Work out the finished part from the listing and answer in its coordinate system (mm). Face numbers are marked on the shaded views. A direction names the side the tool comes from. Give positions to 0.01 mm unless a question says otherwise; leave off trailing zeros. Order: outer loops, then holes, each group sorted by start corner. A loop starts at its lowest first (then second) coordinate and runs counter-clockwise, first axis right, second up.
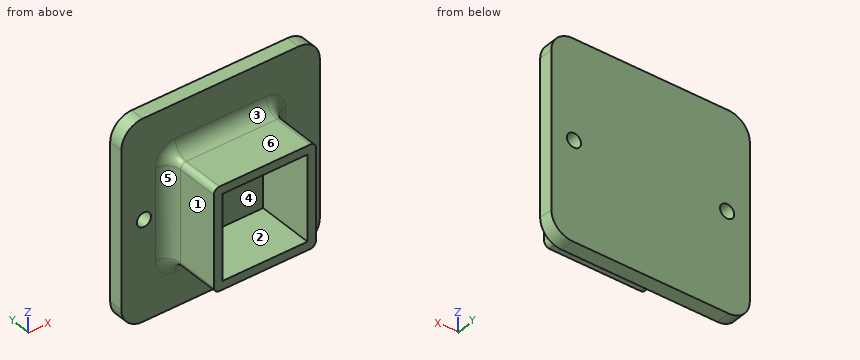
```python
from build123d import *

# Parameters (mm, degrees)
SKETCH1_W           = 36
SKETCH1_H           = 36
SKETCH1_W_2         = 30.02
SKETCH1_H_2         = 30.02
BOSS_EXTRUDE1_DEPTH = 20
SKETCH2_W           = 70
SKETCH2_H           = 70
BOSS_EXTRUDE2_DEPTH = 5
FILLET1_R           = 7.5
SKETCH3_R           = 2.5
CUT_EXTRUDE1_DEPTH  = 56.452682532
FILLET2_R           = 2
FILLET3_R           = 5


with BuildPart() as part:
    # Sketch1 → Boss-Extrude1 (new body)
    with BuildSketch(Plane(origin=(0, 0, 0), x_dir=(1, 0, 0), z_dir=(0, 1, 0))):
        Rectangle(SKETCH1_W, SKETCH1_H)
        Rectangle(SKETCH1_W_2, SKETCH1_H_2, mode=Mode.SUBTRACT)
    extrude(amount=BOSS_EXTRUDE1_DEPTH)

    # Sketch2 → Boss-Extrude2 (add)
    with BuildSketch(Plane(origin=(0, 20, 0), x_dir=(1, 0, 0), z_dir=(0, 1, 0))):
        Rectangle(SKETCH2_W, SKETCH2_H)
    extrude(amount=BOSS_EXTRUDE2_DEPTH)

    # Fillet1
    fillet1_edges = [part.edges().sort_by_distance(p)[0] for p in [
        (35, 22.5, 35),
        (35, 22.5, -35),
        (-35, 22.5, -35),
        (-35, 22.5, 35),
    ]]
    fillet(fillet1_edges, radius=FILLET1_R)

    # Sketch3 → Cut-Extrude1 (cut, through all)
    with BuildSketch(Plane(origin=(0, 25, 0), x_dir=(1, 0, 0), z_dir=(0, 1, 0))):
        with Locations(Location((-27, 0, 0), (0, 0, 270))):
            Circle(SKETCH3_R)
        with Locations(Location((27, 0, 0), (0, 0, 270))):
            Circle(SKETCH3_R)
    extrude(amount=-CUT_EXTRUDE1_DEPTH, mode=Mode.SUBTRACT)

    # Fillet2
    fillet2_edges = [part.edges().sort_by_distance(p)[0] for p in [
        (18, 10, 18),
        (-18, 10, 18),
        (-18, 10, -18),
        (18, 10, -18),
    ]]
    fillet(fillet2_edges, radius=FILLET2_R)

    # Fillet3
    fillet3_edges = [part.edges().sort_by_distance(p)[0] for p in [
        (0, 20, -18),
        (18, 20, 0),
        (0, 20, 18),
        (-18, 20, 0),
        (17.414213562, 20, -17.414213562),
        (17.414213562, 20, 17.414213562),
        (-17.414213562, 20, -17.414213562),
        (-17.414213562, 20, 17.414213562),
    ]]
    fillet(fillet3_edges, radius=FILLET3_R)


solid = part.part
```
1. The part is cut by section D-D (x = 4.5). Write down the section's boundary in (y, z), then the cut area to 3 significant figures.
Findings below:
outline: (0, -18) - (15, -18) arc R5 cw to (20, -23) - (20, -35) - (25, -35) - (25, 35) - (20, 35) - (20, 23) arc R5 cw to (15, 18) - (0, 18) - (0, 15.01) - (20, 15.01) - (20, -15.01) - (0, -15.01) - close
area: 480 mm2
2. Straight lines are drawn through the part: probe 1 along X at (y, z) = (22.65, 0); probe 2 along Z at (x, y) = (-6.5, 4.75). For each, find the intervals that lie inside material, in ascending order.
Findings below:
probe 1: x = -35 to -29.5, -24.5 to 24.5, 29.5 to 35
probe 2: z = -18 to -15.01, 15.01 to 18
3. The mould has two halves that part along Z. Classify the marked faces 1, 2 and 3: pulls with the +Z half, pulls with the -Z half, needs draft (parallel to the pull), parting line crosses it, or undercut.
Findings below:
face 1: needs draft
face 2: undercut
face 3: pulls with the +Z half
4. Which of the six approach directions +Z, -Z, +X, -X, +Y, -Y give full straight-line access (tool end or side, diameter ignored) to the marked faces 4, 5 and 6?
Findings below:
face 4: -Y
face 5: +Z, -Z, -X, -Y
face 6: +Z, +X, -X, -Y
5. The part is cut by section B-B (y = 10.5). Write down the section's boundary in (x, z), then the cut area to 3 significant figures.
Findings below:
outline: (-18, -16) arc R2 ccw to (-16, -18) - (16, -18) arc R2 ccw to (18, -16) - (18, 16) arc R2 ccw to (16, 18) - (-16, 18) arc R2 ccw to (-18, 16) - close; hole (-15.01, -15.01) - (15.01, -15.01) - (15.01, 15.01) - (-15.01, 15.01) - close
area: 391 mm2
6. The part is cut by section A-A (z = 0). Write down the section's boundary in (x, y), then the cut area to 3 significant figures.
Findings below:
outline: (-35, 20) - (-29.5, 20) - (-29.5, 25) - (-35, 25) - close; (-24.5, 20) - (-23, 20) arc R5 cw to (-18, 15) - (-18, 0) - (-15.01, 0) - (-15.01, 20) - (15.01, 20) - (15.01, 0) - (18, 0) - (18, 15) arc R5 cw to (23, 20) - (24.5, 20) - (24.5, 25) - (-24.5, 25) - close; (29.5, 20) - (35, 20) - (35, 25) - (29.5, 25) - close
area: 430 mm2
7. The part is cut by section C-C (z = 10). Write down the section's boundary in (x, y).
Findings below:
outline: (-35, 20) - (-23, 20) arc R5 cw to (-18, 15) - (-18, 0) - (-15.01, 0) - (-15.01, 20) - (15.01, 20) - (15.01, 0) - (18, 0) - (18, 15) arc R5 cw to (23, 20) - (35, 20) - (35, 25) - (-35, 25) - close
8. Given P1, Ø12, axis at x = -1.5, y = 10, coming from the -Z side; P2, Ø10, axis at x = -2, y = 8, coming from the +Z side; P3, Ø4.5, axis at x = 27, z = 0, coming from the +Y side; P4, Ø9, axis at x = -4.5, z = 1, coming from the -Y side, each flat-ended and moving along its own axis, determine where each tip first touches the part or whether it passes through.
Findings below:
P1: stops at z = -18.1
P2: stops at z = 18
P3: passes through
P4: stops at y = 20
